CAD build for the part. Positions are in the model's coordinates, mm. Round coordinates to 2 decimals unless told otherwise and drop trailing zeros. Order: outer loops, then holes, each group sorted by start corner. A loop starts at its lowest first (then second) coordinate and runs counter-clockwise, first axis right, second up. Notation, with made-up numbers: M -19.5,89 L 1.5,89 A27 cw 1.5,114 Z; hole C 23.25,86 d1. An arc over 180 degrees is marked long. Answer as a JSON object with one key per item and string values. Group by question number.
Autodesk Inventor part; units mm, degrees
ref_plane "Начальная плоскость" through (0, 0, 83.8145) normal (0, 0, 1) x (1, 0, 0)
ref_plane "Конечная плоскость" through (0, 0, 661.5924) normal (0, 0, 1) x (1, 0, 0)
ref_plane "РабПлоскость4" through (-8, 209.5676, 565.5202) normal (0, 0.9113542, -0.4116231) x (1, 0, 0)
ref_plane "Начальная плоскость" through (0, 0, 83.8145) normal (0, 0, 1) x (1, 0, 0)
ref_plane "Конечная плоскость" through (0, 0, 661.5924) normal (0, 0, 1) x (1, 0, 0)
sketch "Эскиз" plane through (0, 0, 0) normal (0, 0, 1) x (1, 0, 0)
  circle A0 centre (0, 0) radius 7
  circle A1 centre (0, 0) radius 8
  dimension "d0" = 16
  dimension "d1" = 1
extrude "Тело" add sketch "Эскиз" along normal up to surface (577.7778 mm away) from surface at 83.8145
sketch "Sketch3" plane through (0, 0, 0) normal (0, 0, 1) x (1, 0, 0)
  line L0 (0, 0) -> (10, 0)
ref_plane "Work Plane3" through (0, 0, 0) normal (0, -1, 0) x (1, 0, 0)
sketch "Sketch4" plane through (0, 0, 0) normal (0, -1, 0) x (1, 0, 0)
  line L0 (-2, 83.8145) -> (12, 83.8145)
  line L1 (-2, 661.5924) -> (12, 661.5924)
  dimension "d7" = 577.7778
ref_plane "РабПлоскость4" through (-8, 209.5676, 565.5202) normal (0, 0.9113542, -0.4116231) x (1, 0, 0)
split "Разделение1" plane through (-8, 209.5676, 565.5202) removes the side toward (0, 0.9113542, -0.4116231)
ref_plane "РабПлоскость5" through (57, 468.0246, 446.5907) normal (0, 0.4116231, 0.9113542) x (1, 0, 0)
split "Разделение2" plane through (57, 468.0246, 446.5907) removes the side toward (0, 0.4116231, 0.9113542)
equation "\"d0\" = G_H"
equation "\"d1\" = G_T"
equation "\"d2\" = G_L"
equation "\"G_H\" = 16"
equation "\"G_T\" = 1"
equation "\"G_L\" = d7"
equation "\"G_OFFSET_START\" = -83.81455"
equation "\"G_OFFSET_END\" = -2.19454"
equation "\"d4\" = -G_OFFSET_START"
equation "\"d5\" = G_OFFSET_END + B_L"
equation "\"B_L\" = 663.78693"
properties part number "Труба 16x1-577,78 ГОСТ 10704-91" material "Сталь, мягкая"
Item 1: Cut at B-B, the plane x = -3.25. Give the cut face in (y, z).
Item 2: Two-plate mould, pull along Y, no slides. Class faces 1 (the face through (7.07, 1.22, 104.23)), 2 (the face through (-0.91, -6.94, 369.54)), 3 (the face through (4.301, -6.746, 368.629)): +Y half, -Y half, draft (parallel to the pull), parting line (faces both ways), or undercut.
Item 3: Cut at C-C, the plane z = 380. Give the cut face in (x, y), and give its area (3 significant figures).
Item 4: Flat gauge pins, fed straight in: pin 1 Ø5 at (y, z) = (5, 513) entering from +X; pin 2 Ø6 at (x, z) = (5, 316) entering from -Y; pin 3 Ø8 at (y, z) = (-1.5, 387.5) entering from -X; pin 4 Ø2 at (x, z) = (2.5, 334.5) entering from +Y. Where does each tip first touch, or does it go through?
Item 5: Drill centre lines: line 1 (X direction, y = -1.25, z = 611.5); line 2 (X direction, y = -0.25, z = 622); line 3 (Y direction, x = -0.5, z = 574.5). Where is each one in solid material? Low to high. Write a range as [from, to].
Item 6: Cut at A-A, the plane y = -4.5. Give the cut face in (x, z), and give its area (3 significant figures).
Response values:
{
 "1": {"outline": "M -7.31,85.34 L -6.2,87.8 L -6.2,660.78 L -7.31,661.28 Z; M 6.2,115.25 L 7.31,117.71 L 7.31,654.68 L 6.2,655.18 Z"},
 "2": {"face 1": "+Y half", "face 2": "undercut", "face 3": "parting line"},
 "3": {"outline": "C 0,0 d16; hole C 0,0 d14", "area": "47.1 mm^2"},
 "4": {"pin 1": "x = 7.6", "pin 2": "y = -7.75", "pin 3": "x = -8", "pin 4": "y = 7.86"},
 "5": {"line 1": "[-7.9, -6.89], [6.89, 7.9]", "line 2": "[-8, -7], [7, 8]", "line 3": "[-7.98, -6.98], [6.98, 7.98]"},
 "6": {"outline": "M -6.61,91.56 L -5.36,91.56 L -5.36,660.01 L -6.61,660.01 Z; M 5.36,91.56 L 6.61,91.56 L 6.61,660.01 L 5.36,660.01 Z", "area": "1,420 mm^2"}
}
